Autodesk Inventor part; units mm, degrees
ref_plane "YZ Plane" through (0, 0, 0) normal (1, 0, 0) x (0, 1, 0)
ref_plane "XZ Plane" through (0, 0, 0) normal (0, 1, 0) x (-1, 0, 0)
ref_plane "XY Plane" through (0, 0, 0) normal (0, 0, 1) x (1, 0, 0)
sketch "Sketch1" plane through (0, 0, 0) normal (0, 0, 1) x (1, 0, 0)
  line L0 (-5.3, 15) -> (-20.5165, 15)
  line L1 (-4.6, 15.7) -> (-5.3, 15)
  line L2 (4.6, 15.7) -> (-4.6, 15.7)
  line L3 (5.3, 15) -> (4.6, 15.7)
  line L4 (20.5165, 15) -> (5.3, 15)
  line L5 (21.5, 14.0165) -> (20.5165, 15)
  line L6 (21.5, -8) -> (21.5, 14.0165)
  line L7 (20, -9.5) -> (21.5, -8)
  line L8 (9.45, -9.5) -> (20, -9.5)
  line L9 (6.6, -6.65) -> (9.45, -9.5)
  line L10 (6.6, -4.35) -> (6.6, -6.65)
  line L11 (7.7, -3.25) -> (6.6, -4.35)
  arc A0 (9.6, -1.075) -> (7.7, -3.25) centre (9.8292, -3.1926) ccw
  line L12 (10, -0.675) -> (9.6, -1.075)
  line L13 (10, 0.675) -> (10, -0.675)
  line L14 (9.6, 1.075) -> (10, 0.675)
  arc A1 (7.7, 3.1) -> (9.6, 1.075) centre (9.828, 3.1928) ccw
  line L15 (7.3, 3.5) -> (7.7, 3.1)
  line L16 (-7.3, 3.5) -> (7.3, 3.5)
  line L17 (-7.7, 3.1) -> (-7.3, 3.5)
  arc A2 (-9.6, 1.075) -> (-7.7, 3.1) centre (-9.828, 3.1928) ccw
  line L18 (-10, 0.675) -> (-9.6, 1.075)
  line L19 (-10, -0.675) -> (-10, 0.675)
  line L20 (-9.6, -1.075) -> (-10, -0.675)
  arc A3 (-7.7, -3.25) -> (-9.6, -1.075) centre (-9.8292, -3.1926) ccw
  line L21 (-6.6, -4.35) -> (-7.7, -3.25)
  line L22 (-6.6, -6.65) -> (-6.6, -4.35)
  line L23 (-9.45, -9.5) -> (-6.6, -6.65)
  line L24 (-20, -9.5) -> (-9.45, -9.5)
  line L25 (-21.5, -8) -> (-20, -9.5)
  line L26 (-21.5, 14.0165) -> (-21.5, -8)
  line L27 (-20.5165, 15) -> (-21.5, 14.0165)
  point P0 (0, 0)
  point P1 (0, 0)
extrude "Extrusion1" add sketch "Sketch1" along normal blind 10
sketch "Sketch2" plane through (-21.5, -8, 0) normal (-1, 0, 0) x (0, 0, 1)
  line L0 (0, 22.0165) -> (0, 0)
  line L1 (0, 0) -> (10, 0)
  line L2 (10, 22.0165) -> (10, 0)
  line L3 (0, 22.0165) -> (10, 22.0165)
  line L4 (10, 0) -> (10, 22.0165)
  line L5 (0, 22.0165) -> (10, 22.0165)
  line L6 (0, 0) -> (0, 22.0165)
  line L7 (0, 0) -> (10, 0)
  circle A0 centre (4, 18) radius 2.5
  point P0 (0, 8)
extrude "Extrusion2" cut sketch "Sketch2" against normal blind 6.7 contours A0
mirror "Mirror1" about plane through (0, 0, 0) normal (1, 0, 0) of "Extrusion2"
sketch "Sketch3" plane through (-4.6, 15.7, 0) normal (0, 1, 0) x (1, 0, 0)
  line L0 (9.2, 0) -> (0, 0)
  line L1 (0, 0) -> (0, -10)
  line L2 (9.2, -10) -> (0, -10)
  line L3 (9.2, 0) -> (9.2, -10)
  line L4 (0, -10) -> (9.2, -10)
  line L5 (9.2, 0) -> (9.2, -10)
  line L6 (0, 0) -> (9.2, 0)
  line L7 (0, 0) -> (0, -10)
  circle A0 centre (4.6, -5) radius 3.65
  point P0 (4.6, 0)
extrude "Extrusion3" cut sketch "Sketch3" against normal blind 2 contours A0
properties part number "HGR20B"
Design review of the part built by this model. Coordinates are the model's own, in mm. A direction names the side the tool comes from. Give positions to 0.01 mm unless a question says otherwise; leave off trailing zeros. Loops run counter-clockwise (first coordinate to the right, second up) from the corner with the lowest first, then second, coordinate; pieces in that order, holes last. Notation, with made-up numbers: M 89.25,-18 L 108.25,-18 A21 cw 108.25,16 Z; hole C -36,62 d8. An arc over 180 degrees is marked long. One line per question, with ' | ' between items. Start each with the question number.
1. Add section D-D (x = -10.5). Write out the cut boundary in (y, z).
2. The part is to be moulded in two halves that separate along Z. For faces 1 (the face through (-15, -9.5, 5)), 2 (the face through (0, 6, 10)), 3 (the face through (-18.2, 7.56, 3.46)), 4 (the face through (0, 6, 0)), say which applies: released by +Z, released by -Z, zero draft, split by the parting line, or undercut.
3. Add section C-C (x = 0). Write out the cut boundary in (y, z).
4. For faces 5 (the face through (0, 13.7, 5)), 6 (the face through (-14.8, 10, 4)), 7 (the face through (6.6, -5, 5)), 8 (the face through (8.21, -1.81, 4.93)), 9 (the face through (14.8, 10, 4)), list the 3-axis set-ups (+Z, -Z, +X, -X, +Y, -Y) from which the entire face can be reached by the end or side of a thin tool; tool diameter is ignored.
5. Add section A-A (y = 10). Write out the cut boundary in (x, z).
6. To check wall thickness, follow L1, parallel to Y at x = -16.5, z = 4; L2, parallel to X at y = -5.5, z = 4.5; L3, parallel to Y at x = -5.5, z = 9.25. State the ranges of each line that lie inside material, in increasing order.
7. Insertion check: P1, Ø2, axis at x = -1.5, z = 4.5, coming from the +Y side; P2, Ø5, axis at x = -14, z = 5, coming from the +Y side; P3, Ø3, axis at y = 10, z = 4, coming from the +X side. Each pin has a flat end and moves straight along its axis. Give the tip position at first contact, or say it passes through.
Worked out:
1) outline: M -9.5,0 L 15,0 L 15,10 L -9.5,10 Z
2) face 1: zero draft | face 2: released by +Z | face 3: undercut | face 4: released by -Z
3) outline: M 3.5,0 L 15.7,0 L 15.7,1.35 L 13.7,1.35 L 13.7,8.65 L 15.7,8.65 L 15.7,10 L 3.5,10 Z
4) face 5: +Y | face 6: -X | face 7: +Z, -Z, -Y | face 8: +Z, -Z | face 9: +X
5) outline: M -21.5,0 L 21.5,0 L 21.5,1.5 L 14.8,1.5 L 14.8,6.5 L 21.5,6.5 L 21.5,10 L -21.5,10 L -21.5,6.5 L -14.8,6.5 L -14.8,1.5 L -21.5,1.5 Z
6) L1: y = -9.5 to 7.5, 12.5 to 15 | L2: x = -21.5 to -6.6, 6.6 to 21.5 | L3: y = 3.5 to 15
7) P1: stops at y = 13.7 | P2: stops at y = 15 | P3: stops at x = 14.8
